Verification items for this drawing (mm, ordinates from the low corner). Coordinates: 2 decimals unless noted, no trailing zeros. Order: outer loops, then holes, each group sorted by start corner. A loop starts at its lowest first (then second) coordinate and runs counter-clockwise, first axis right, second up.
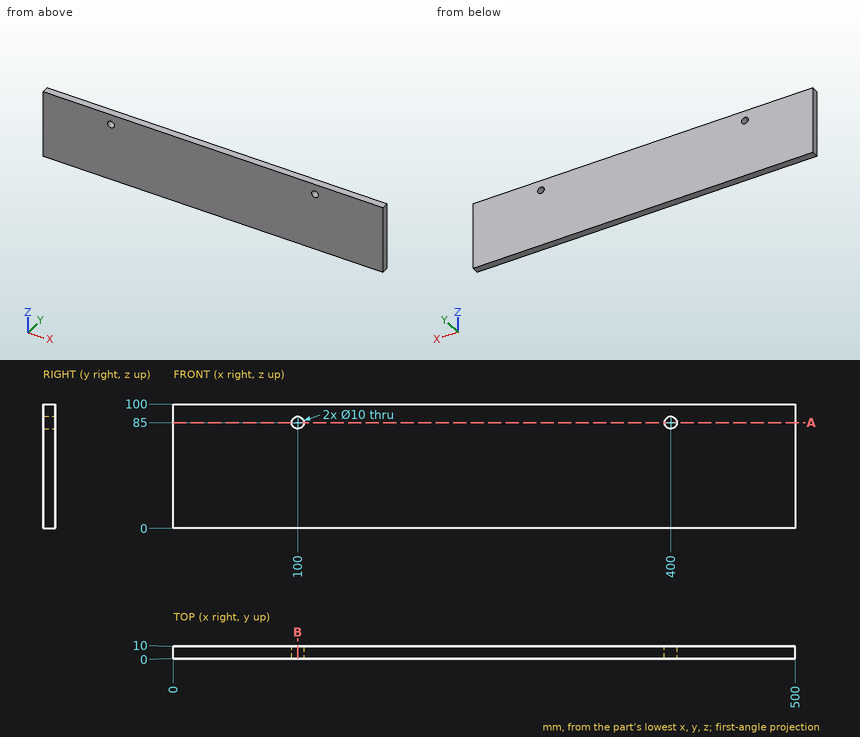
Item 1: Thickness scan on line 1 along X through (y, z) = (8.25, 85); line 2 along X through (y, z) = (0.75, 82). Record the ranges inside material, lowest first.
Item 2: Sectioned sample at B-B (x = 100). Record the cut outline in (y, z).
Item 3: Sectioned sample at A-A (z = 85). Record the cut outline in (x, y), and give its area (3 significant figures).
Item 4: Depth check by flat-ended pin: P1, Ø8, axis at x = 100, z = 85, coming from the +Y side. Enter the tip coordinate at first touch or a pass-through.
Geometry check:
1. line 1: x = 0 to 95, 105 to 395, 405 to 500
1. line 2: x = 0 to 96, 104 to 396, 404 to 500
2. outline: (0, 0) - (10, 0) - (10, 80) - (0, 80) - close; (0, 90) - (10, 90) - (10, 100) - (0, 100) - close
3. outline: (0, 0) - (95, 0) - (95, 10) - (0, 10) - close; (105, 0) - (395, 0) - (395, 10) - (105, 10) - close; (405, 0) - (500, 0) - (500, 10) - (405, 10) - close
3. area: 4,800 mm2
4. P1: passes through
